For this review, take the finished solid that the model builds, in its own axes (mm). Face numbers are marked on the shaded views. A direction names the side the tool comes from. Coordinates: 2 decimals unless noted, no trailing zeros. Loops run counter-clockwise (first coordinate to the right, second up) from the corner with the lowest first, then second, coordinate; pieces in that order, holes last. Notation, with made-up numbers: (22, -33.5) -> (38, -33.5) arc R11 cw to (38, -20.5) -> close; hole circle Ø1 at (88.25, -9). An arc over 180 degrees is marked (long way). One line per item, written item: value.
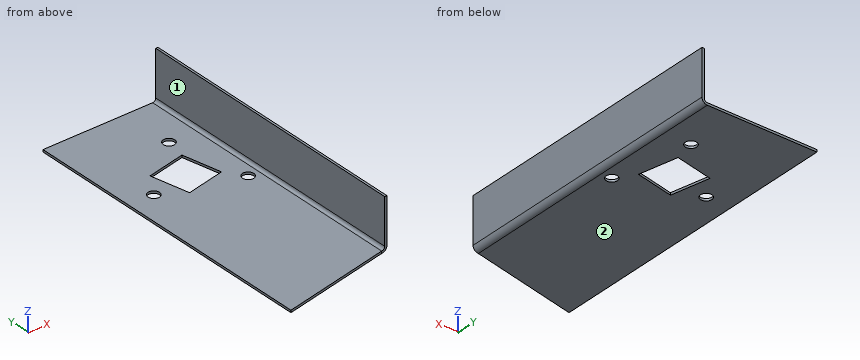
Autodesk Inventor part; units mm, degrees
ref_plane "YZ Plane" through (0, 0, 0) normal (1, 0, 0) x (0, 1, 0)
ref_plane "XZ Plane" through (0, 0, 0) normal (0, 1, 0) x (-1, 0, 0)
ref_plane "XY Plane" through (0, 0, 0) normal (0, 0, 1) x (1, 0, 0)
sketch "Sketch1" plane through (0, 0, 0) normal (0, 0, 1) x (1, 0, 0)
  line L0 (-51, 125) -> (51, 125)
  line L1 (51, 125) -> (51, -125)
  line L2 (51, -125) -> (-51, -125)
  line L3 (-51, -125) -> (-51, 125)
  line L4 (-51, 125) -> (51, -125) construction
  point P0 (0, 0)
  point P1 (0, 0)
  dimension "d0" = 102
  dimension "d1" = 250
extrude "Plate1" add sketch "Sketch1" along normal blind 2
sketch "Sketch4" plane through (49, 125, 0) normal (1, 0, 0) x (0, 1, 0)
  line L0 (-250, 0) -> (0, 0)
  line L1 (0, 0) -> (0, 45)
  line L2 (0, 45) -> (-250, 45)
  line L3 (-250, 45) -> (-250, 0)
edge flange "Flange1" height 45 angle 90 thickness 2 bend radius 2.75 thickness toward (1, 0, 0) relief round relief width 2 relief depth 1 edges at (51, 0, 2) wall of the first edge with corners at (49, -125, 0) (49, 125, 0) (49, 125, 45) (49, -125, 45)
bend "Bend1"
corner "Corner1"
sketch "Sketch5" plane through (0, 0, 0) normal (0, 0, -1) x (-1, 0, 0)
  line L0 (-46.25, 125) -> (-46.25, -125)
  line L1 (51, -125) -> (-46.25, -125)
  line L2 (51, 125) -> (51, -125)
  line L3 (-46.25, 125) -> (51, 125)
  line L4 (51, -125) -> (51, -145.6711)
  line L5 (-46.25, -125) -> (51, -125)
  line L6 (51, -145.6711) -> (-46.25, -125)
  point P0 (0, 0)
  dimension "d25" = 12
extrude "Extrusion2" add sketch "Sketch5" against normal up to surface (2 mm away) contours L1 L4 L6
sketch "Sketch7" plane through (0, 0, 0) normal (0, 0, 1) x (1, 0, 0)
  line L0 (46.25, -125) -> (-51, -145.6711)
  circle A0 centre (36.9805, 9.3484) radius 5.05
  line L1 (36.9805, 9.3484) -> (22.4267, 77.8187) construction
  line L2 (26.006, 24.9066) -> (18.7291, 59.1418)
  circle A1 centre (22.4267, 77.8187) radius 5.05
  line L3 (-28.9852, 31.1089) -> (36.9805, 9.3484) construction
  line L4 (26.006, 24.9066) -> (-15.5061, 51.8649) construction
  line L5 (18.7291, 59.1418) -> (-15.5061, 51.8649)
  line L6 (-8.2292, 17.6297) -> (26.006, 24.9066)
  line L7 (18.7291, 59.1418) -> (-8.2292, 17.6297) construction
  line L8 (-15.5061, 51.8649) -> (-8.2292, 17.6297)
  line L9 (22.3675, 42.0242) -> (-28.9852, 31.1089) construction
  line L10 (22.4267, 77.8187) -> (-28.9852, 31.1089) construction
  circle A2 centre (-28.9852, 31.1089) radius 5.05
  point P0 (0, 0)
  point P1 (-47.5274, -178.5141)
  point P2 (5.2499, 38.3858)
  point P3 (-51, -145.6711)
  dimension "d32" = 35
  dimension "d33" = 35
  dimension "d34" = 10.1
  dimension "d35" = 70
  dimension "d36" = 60
  dimension "d37" = 25
extrude "Extrusion3" cut sketch "Sketch7" along normal through all
equation "\"d33\" = d32"
equation "\"d2\" = Thickness"
equation "\"d15\" = BendReliefWidth"
equation "\"d16\" = BendReliefDepth"
equation "\"d17\" = MinimumRemnant"
equation "\"d18\" = TransitionRadius"
equation "\"d21\" = BendRadius"
equation "\"d22\" = CornerReliefSize"
equation "\"d23\" = GapSize"
equation "\"d24\" = JacobiRadiusSize"
equation "\"BendReliefWidth\" = Thickness"
equation "\"BendReliefDepth\" = 0.5 * Thickness"
equation "\"CornerReliefSize\" = 4 * Thickness"
equation "\"MinimumRemnant\" = 2 * Thickness"
equation "\"TransitionRadius\" = BendRadius"
equation "\"JacobiRadiusSize\" = BendRadius"
equation "\"GapSize\" = Thickness"
properties part number "MNT-CDF-613 big way" material "Stainless Steel"
1. Insertion check: pin 1 Ø5 at (x, z) = (48, 25) entering from -Y; pin 2 Ø2 at (x, y) = (38, -108) entering from +Z; pin 3 Ø8 at (x, y) = (36.98, 9.35) entering from -Z. Each pin has a flat end and moves straight along its axis. Give the tip position at first contact, or say it passes through.
Return value:
pin 1: stops at y = -125
pin 2: stops at z = 2
pin 3: passes through
2. Take a section at B-B, the plane x = -4.5. Give the boundary of the cut face in (y, z), and give its area (3 significant figures).
Return value:
outline: (-135.79, 0) -> (18.42, 0) -> (18.42, 2) -> (-135.79, 2) -> close; (54.2, 0) -> (125, 0) -> (125, 2) -> (54.2, 2) -> close
area: 450 mm2
3. Take a section at A-A, the plane y = -47.5. Give the boundary of the cut face in (x, z).
Return value:
outline: (-51, 0) -> (46.25, 0) arc R4.75 ccw to (51, 4.75) -> (51, 45) -> (49, 45) -> (49, 4.75) arc R2.75 cw to (46.25, 2) -> (-51, 2) -> close
4. For the marked faces 1 and 2, list the 3-axis set-ups (+Z, -Z, +X, -X, +Y, -Y) from which the entire face can be reached by the end or side of a thin tool; tool diameter is ignored.
Return value:
face 1: +Z, -X, +Y, -Y
face 2: -Z, +X, -X, +Y, -Y
5. Take a section at C-C, the plane y = 20.5. Give the boundary of the cut face in (x, z), and give its area (3 significant figures).
Return value:
outline: (-51, 0) -> (-8.84, 0) -> (-8.84, 2) -> (-51, 2) -> close; (5.27, 0) -> (46.25, 0) arc R4.75 ccw to (51, 4.75) -> (51, 45) -> (49, 45) -> (49, 4.75) arc R2.75 cw to (46.25, 2) -> (5.27, 2) -> close
area: 259 mm2
6. To check wall thickness, follow probe 1 along Z at (x, y) = (-22.5, 113.5); probe 2 along X at (y, z) = (-11, 20); probe 3 along X at (y, z) = (-76, 3). State the ranges of each line that lie inside material, in increasing order. Write a range as from..to.
Return value:
probe 1: z = 0..2
probe 2: x = 49..51
probe 3: x = 48.37..50.67
7. Take a section at D-D, the plane z = 9. Give the boundary of the cut face in (x, y).
Return value:
outline: (49, -125) -> (51, -125) -> (51, 125) -> (49, 125) -> close
